Geometry: final body of the model. Coordinates: model frame, mm. A direction names the side the tool comes from. Give positions to 0.01 mm unless a question says otherwise; leave off trailing zeros. Write each loop counter-clockwise with the first axis right and the second up, starting at its lowest first coordinate (ties: lowest second). Pieces come first, ordered by that corner, then holes. Notation, with made-up numbers: (22, -35.5) -> (80, -35.5) arc R19 ccw to (80, -21.5) -> close; hole circle Ø1 at (-2.5, -37). An arc over 180 degrees is marked (long way). Answer in a Markdown table with one row per item. Add a question column.
Item 1: Section query B-B on x = -139. Output: boundary loops of the cut face in (y, z), plus the area to 3 significant figures.
Item 2: Section query C-C on y = 130. State how many separate pieces and enclosed holes the cut face has, plus the area to 3 significant figures.
Item 3: Section query A-A on z = 0. Output: boundary loops of the cut face in (x, y), plus the area to 3 significant figures.
Item 4: Draft query along Y for faces 1 (the flat face through (-274, 400, 116)), 2 (the conical face through (-9.4, -33.2, -105.5)), 3 (the cylindrical face through (-293.856, 379.72, -124.255)), 4 (the flat face through (-533, 360, -83)). Return one class per face: +Y half, -Y half, draft (parallel to the pull), parting line (faces both ways), or undercut.
Item 5: Access query for faces 5 (the cylindrical face through (-512.288, 405.07, 141.49)), 6 (the cylindrical face through (-80.98, 107.384, 23.846)), 7 (the flat face through (-50, 123, 83)), 8 (the flat face through (-25, 180, 2)). Directions: +Z, -Z, +X, -X, +Y, -Y. A direction counts if a zero-diameter tool reaches every point of the face in a straight line with its end or side. Return the directions, or none.
Item 6: First-contact query: P1, Ø8, axis at x = -285, y = 0, coming from the -Z side; P2, Ø24, axis at x = -540, z = -130, coming from the -Y side; P3, Ø10, axis at x = -452.5, z = -1.5, coming from the -Y side; P4, Ø8, axis at x = -249, y = 145, coming from the -Z side. Flat tips, straight axial feed; report the tip coordinate or a pass-through.
Item 7: Material intervals for probe 1 along X at (y, z) = (370, 130); probe 2 along Y at (x, z) = (-23, -130); probe 3 along X at (y, z) = (403.5, -130), sorted ascending. Write a range as from..to.
```python
from build123d import *

# Parameters (mm, degrees)
SKETCH2_R                                           = 145
SKETCH2_R_2                                         = 110
BOSS_EXTRUDE2_START                                 = -50
SKETCH8_W                                           = 360
SKETCH8_H                                           = 360
SKETCH8_R                                           = 145
BOSS_EXTRUDE2_DEPTH                                 = 50
FILLET1_R                                           = 20
CBORE_FOR_0_BINDING_HEAD_MACHINE_SCREW3_D           = 29.999999944
CBORE_FOR_0_BINDING_HEAD_MACHINE_SCREW3_DEPTH       = 50
CBORE_FOR_0_BINDING_HEAD_MACHINE_SCREW3_CBORE_D     = 59.999999888
CBORE_FOR_0_BINDING_HEAD_MACHINE_SCREW3_CBORE_DEPTH = 10.000000066
SKETCH21_W                                          = 360
SKETCH21_H                                          = 360
SKETCH21_R                                          = 145
BOSS_EXTRUDE4_DEPTH                                 = 50
CBORE_FOR_0_BINDING_HEAD_MACHINE_SCREW5_D           = 29.999999944
CBORE_FOR_0_BINDING_HEAD_MACHINE_SCREW5_DEPTH       = 50
CBORE_FOR_0_BINDING_HEAD_MACHINE_SCREW5_CBORE_D     = 59.999999888
CBORE_FOR_0_BINDING_HEAD_MACHINE_SCREW5_CBORE_DEPTH = 10.000000066
FILLET2_R                                           = 20
CHAMFER1_SIZE                                       = 10


with BuildPart() as part:
    # Sweep12: sweep along a path in Sketch1
    with BuildLine(Plane.XY) as sweep12_path:
        Line((0, 0), (-150, 0))
        ThreePointArc((-150, 0), (-333.847763109, 76.152236891), (-410, 260))
        Line((-410, 260), (-410, 410))
    # Sketch2 → Sweep12 (sweep)
    with BuildSketch(Plane(origin=(0, 0, 0), x_dir=(0, 0, -1), z_dir=(1, 0, 0))):
        Circle(SKETCH2_R)
        Circle(SKETCH2_R_2, mode=Mode.SUBTRACT)
    sweep(path=sweep12_path.line)

    # Sketch8 → Boss-Extrude2 (add)
    with BuildSketch(Plane(origin=(0, 0, 0), x_dir=(0, 0, -1), z_dir=(1, 0, 0)).offset(BOSS_EXTRUDE2_START)):
        Rectangle(SKETCH8_W, SKETCH8_H)
        with Locations(Location((0, 0, 0), (0, 0, 270))):
            Circle(SKETCH8_R, mode=Mode.SUBTRACT)
    extrude(amount=BOSS_EXTRUDE2_DEPTH)

    # Fillet1
    fillet1_edges = [part.edges().sort_by_distance(p)[0] for p in [
        (-25, 180, -180),
        (-25, -180, -180),
        (-25, -180, 180),
        (-25, 180, 180),
    ]]
    fillet(fillet1_edges, radius=FILLET1_R)

    # CBORE for #0 Binding Head Machine Screw3
    with Locations(Plane(origin=(0, 0, 0), x_dir=(0, 0, -1), z_dir=(1, 0, 0))):
        with Locations((-130, 130), (130, 130), (130, -130), (-130, -130)):
            CounterBoreHole(CBORE_FOR_0_BINDING_HEAD_MACHINE_SCREW3_D / 2, CBORE_FOR_0_BINDING_HEAD_MACHINE_SCREW3_CBORE_D / 2, CBORE_FOR_0_BINDING_HEAD_MACHINE_SCREW3_CBORE_DEPTH, depth=CBORE_FOR_0_BINDING_HEAD_MACHINE_SCREW3_DEPTH)

    # Sketch21 → Boss-Extrude4 (add)
    with BuildSketch(Plane(origin=(0, 410, 0), x_dir=(1, 0, 0), z_dir=(0, 1, 0))):
        with Locations((-410, 0)):
            Rectangle(SKETCH21_W, SKETCH21_H)
        with Locations(Location((-410, 0, 0), (0, 0, 180))):
            Circle(SKETCH21_R, mode=Mode.SUBTRACT)
    extrude(amount=-BOSS_EXTRUDE4_DEPTH)

    # CBORE for #0 Binding Head Machine Screw5
    with Locations(Plane(origin=(0, 410, 0), x_dir=(1, 0, 0), z_dir=(0, 1, 0))):
        with Locations((-540, 130), (-280, 130), (-280, -130), (-540, -130)):
            CounterBoreHole(CBORE_FOR_0_BINDING_HEAD_MACHINE_SCREW5_D / 2, CBORE_FOR_0_BINDING_HEAD_MACHINE_SCREW5_CBORE_D / 2, CBORE_FOR_0_BINDING_HEAD_MACHINE_SCREW5_CBORE_DEPTH, depth=CBORE_FOR_0_BINDING_HEAD_MACHINE_SCREW5_DEPTH)

    # Fillet2
    fillet2_edges = [part.edges().sort_by_distance(p)[0] for p in [
        (-230, 385, -180),
        (-230, 385, 180),
        (-590, 385, 180),
        (-590, 385, -180),
    ]]
    fillet(fillet2_edges, radius=FILLET2_R)

    # Chamfer1
    chamfer1_edges = [part.edges().sort_by_distance(p)[0] for p in [
        (-410, 410, 110),
        (0, 0, 110),
    ]]
    chamfer(chamfer1_edges, length=CHAMFER1_SIZE)


solid = part.part
```
Findings below:
| question | item | result |
|---|---|---|
| 1 | outline | circle Ø290 at (0, 0); hole circle Ø220 at (0, 0) |
| 1 | area | 28,000 mm^2 |
| 2 | separate pieces | 3 |
| 2 | enclosed holes | 1 |
| 2 | area | 67,200 mm^2 |
| 3 | outline | (-590, 360) -> (-555, 360) -> (-555, 260) arc R405 ccw to (-150, -145) -> (-50, -145) -> (-50, -180) -> (0, -180) -> (0, -120) -> (-10, -110) -> (-150, -110) arc R370 cw to (-520, 260) -> (-520, 400) -> (-530, 410) -> (-590, 410) -> close; (-300, 260) arc R150 ccw to (-150, 110) -> (-10, 110) -> (0, 120) -> (0, 180) -> (-50, 180) -> (-50, 145) -> (-150, 145) arc R115 cw to (-265, 260) -> (-265, 360) -> (-230, 360) -> (-230, 410) -> (-290, 410) -> (-300, 400) -> close |
| 3 | area | 56,400 mm^2 |
| 4 | face 1 | +Y half |
| 4 | face 2 | undercut |
| 4 | face 3 | draft |
| 4 | face 4 | undercut |
| 5 | face 5 | +Y |
| 5 | face 6 | +X |
| 5 | face 7 | none |
| 5 | face 8 | +Z, -Z, +X, +Y |
| 6 | P1 | stops at z = -142.08 |
| 6 | P2 | passes through |
| 6 | P3 | stops at y = -14.8 |
| 6 | P4 | stops at z = -100.77 |
| 7 | probe 1 | x = -590..-555, -525..-295, -265..-230 |
| 7 | probe 2 | y = -180..-145, -115..115, 145..180 |
| 7 | probe 3 | x = -590..-570, -510..-310, -250..-230 |
